from build123d import *
from build123d.topology import SkipClean

# Parameters (mm, degrees)
SKETCH1_R               = 7.9
BOSS_EXTRUDE1_DEPTH     = 1.2
SKETCH2_R               = 1.8
BOSS_EXTRUDE2_DEPTH     = 1.7
CUT_EXTRUDE1_DEPTH      = 12.542530052
CUT_EXTRUDE1_DEPTH_BACK = 12.542530052
SKETCH3_R               = 1.1
BOSS_EXTRUDE3_START     = 2
BOSS_EXTRUDE3_DEPTH     = 2
CUT_EXTRUDE2_DEPTH      = 0.2
CIRPATTERN1_COUNT       = 4
SKETCH6_R               = 1.7
SKETCH6_R_2             = 1.1
BOSS_EXTRUDE4_DEPTH     = 2


with BuildPart() as part:
    # Sketch1 → Boss-Extrude1 (new body)
    with BuildSketch(Plane(origin=(0, 0, 0), x_dir=(1, 0, 0), z_dir=(0, 1, 0))):
        with Locations(Location((0, 0, 0), (0, 0, 270))):
            Circle(SKETCH1_R)
    extrude(amount=BOSS_EXTRUDE1_DEPTH)

    # Sketch2 → Boss-Extrude2 (add)
    with BuildSketch(Plane(origin=(0, 1.2, 0), x_dir=(1, 0, 0), z_dir=(0, 1, 0))):
        with Locations(Location((0, 0, 0), (0, 0, 270))):
            Circle(SKETCH2_R)
    extrude(amount=BOSS_EXTRUDE2_DEPTH)

    # Sketch3 → Cut-Extrude1 (cut, two sides: drawn at the far end of the back side and taken through both)
    with BuildSketch(Plane(origin=(0, 2.9, 0), x_dir=(1, 0, 0), z_dir=(0, 1, 0)).offset(-CUT_EXTRUDE1_DEPTH_BACK)):
        with Locations(Location((0, 0, 0), (0, 0, 270))):
            Circle(SKETCH3_R)
    extrude(amount=CUT_EXTRUDE1_DEPTH + CUT_EXTRUDE1_DEPTH_BACK, mode=Mode.SUBTRACT)

    # Sketch4 → Boss-Extrude3 (add)
    with SkipClean():  # the faces are left unmerged after this step: merging them gives an invalid solid
        with BuildSketch(Plane.XZ.offset(BOSS_EXTRUDE3_START)):
            with BuildLine():
                Line((4.244666906, -6.662792422), (2.951034003, -5.903507289))
                ThreePointArc((2.951034003, -5.903507289), (0, -6.6), (-2.951034003, -5.903507289))
                Line((-2.951034003, -5.903507289), (-4.244666906, -6.662792422))
                ThreePointArc((-4.244666906, -6.662792422), (0, -7.9), (4.244666906, -6.662792422))
            make_face()
        boss_extrude3 = extrude(amount=-BOSS_EXTRUDE3_DEPTH)

    # Sketch5 → Cut-Extrude2 (cut)
    with SkipClean():  # the faces are left unmerged after this step: merging them gives an invalid solid
        with BuildSketch(Plane.XZ.offset(2)):
            with BuildLine():
                Line((-4.050265696, -6.54869054), (-4.244666906, -6.662792422))
                ThreePointArc((-4.244666906, -6.662792422), (0, -7.9), (4.244666906, -6.662792422))
                Line((4.244666906, -6.662792422), (4.050265696, -6.54869054))
                ThreePointArc((4.050265696, -6.54869054), (0, -7.7), (-4.050265696, -6.54869054))
            make_face()
        cut_extrude2 = extrude(amount=-CUT_EXTRUDE2_DEPTH, mode=Mode.SUBTRACT)

    # CirPattern1: Boss-Extrude3, Cut-Extrude2 ×4 about axis
    with SkipClean():  # the faces are left unmerged after this step: merging them gives an invalid solid
        cirpattern1_axis = Axis((0, 0, 0), (0, 1, 0))
        add([boss_extrude3.rotate(cirpattern1_axis, i * 360 / CIRPATTERN1_COUNT) for i in range(1, CIRPATTERN1_COUNT)])
        add([cut_extrude2.rotate(cirpattern1_axis, i * 360 / CIRPATTERN1_COUNT) for i in range(1, CIRPATTERN1_COUNT)], mode=Mode.SUBTRACT)

    # Sketch6 → Boss-Extrude4 (add)
    with SkipClean():  # the faces are left unmerged after this step: merging them gives an invalid solid
        with BuildSketch(Plane.XZ):
            with Locations(Location((0, 0, 0), (0, 0, 90))):
                Circle(SKETCH6_R)
            with Locations(Location((0, 0, 0), (0, 0, 90))):
                Circle(SKETCH6_R_2, mode=Mode.SUBTRACT)
        extrude(amount=BOSS_EXTRUDE4_DEPTH)


solid = part.part
Build history of the part. All positions in model axes, mm. A direction names the side the tool comes from. Round coordinates to 2 decimals unless told otherwise and drop trailing zeros. Write each loop counter-clockwise with the first axis right and the second up, starting at its lowest first coordinate (ties: lowest second). Pieces come first, ordered by that corner, then holes. Notation, with made-up numbers: M 19,70.5 L 61,70.5 A28 cw 61,102.5 Z; hole C -33.75,30 d6. An arc over 180 degrees is marked long. Use CSV: the item, a comma, the result in double quotes.
1. Flat gauge pins, fed straight in: pin 1 (1.5 mm diameter, centred on x = 1, y = 1.5, fed in from -Z); pin 2 (1.8 mm diameter, centred on x = 0, z = 0, fed in from -Y); pin 3 (1 mm diameter, centred on x = 6, z = 5, fed in from -Y). Where does each tip first touch, or does it go through?
Reply:
pin 1,"stops at z = -7.89"
pin 2,"passes through"
pin 3,"stops at y = 0"
2. Saw through at D-D (y = 0.85). Give the cut face in (x, z), plus the area to 3 significant figures.
Reply:
outline,"C 0,0 d15.8; hole C 0,0 d2.2"
area,"192 mm²"
3. Wall check: probe 1 along X at (y, z) = (0.9, 0); probe 2 along X at (y, z) = (-0.85, -0.25); probe 3 along Y at (x, z) = (5.5, 2.75). Give the ranges that are in metal, low to high. Write a range as from..to.
Reply:
probe 1,"x = -7.9..-1.1, 1.1..7.9"
probe 2,"x = -7.9..-6.6, -1.68..-1.07, 1.07..1.68, 6.6..7.9"
probe 3,"y = 0..1.2"
4. Saw through at B-B (z = 0). Give the cut face in (x, y).
Reply:
outline,"M -7.9,-1.8 L -7.7,-1.8 L -7.7,-2 L -6.6,-2 L -6.6,0 L -1.7,0 L -1.7,-2 L -1.1,-2 L -1.1,2.9 L -1.8,2.9 L -1.8,1.2 L -7.9,1.2 Z; M 1.1,-2 L 1.7,-2 L 1.7,0 L 6.6,0 L 6.6,-2 L 7.7,-2 L 7.7,-1.8 L 7.9,-1.8 L 7.9,1.2 L 1.8,1.2 L 1.8,2.9 L 1.1,2.9 Z"
5. Two-plate mould, pull along Y, no slides. Class faces 1 (the face through (1, 2.9, 1)), 2 (the face through (0, -2, 7)), 3 (the face through (-6.28, -1.01, 3.59)): +Y half, -Y half, draft (parallel to the pull), parting line (faces both ways), or undercut.
Reply:
face 1,"+Y half"
face 2,"-Y half"
face 3,"draft"
6. Tool access for faces 4 (the face through (-6.6, -1, 0)), 5 (the face through (6.28, -1.01, -3.59)), 6 (the face through (3.59, -1.01, 6.28)): list every direction of +Z, -Z, +X, -X, +Y, -Y with a clear straight run to the whole face (end or side of a thin tool).
Reply:
face 4,"-Y"
face 5,"-Z, -Y"
face 6,"+X, -Y"
7. Saw through at A-A (y = -0.7). Give the cut face in (x, z).
Reply:
outline,"M -6.66,-4.24 L -5.9,-2.95 A6.6 cw -5.9,2.95 L -6.66,4.24 A7.9 ccw Z; M -4.24,-6.66 A7.9 ccw 4.24,-6.66 L 2.95,-5.9 A6.6 cw -2.95,-5.9 Z; M -4.24,6.66 L -2.95,5.9 A6.6 cw 2.95,5.9 L 4.24,6.66 A7.9 ccw Z; C 0,0 d3.4; M 5.9,-2.95 L 6.66,-4.24 A7.9 ccw 6.66,4.24 L 5.9,2.95 A6.6 cw Z; hole C 0,0 d2.2"
8. Saw through at C-C (x = 0). Give the cut face in (y, z).
Reply:
outline,"M -2,-7.7 L -1.8,-7.7 L -1.8,-7.9 L 1.2,-7.9 L 1.2,-1.8 L 2.9,-1.8 L 2.9,-1.1 L -2,-1.1 L -2,-1.7 L 0,-1.7 L 0,-6.6 L -2,-6.6 Z; M -2,1.1 L 2.9,1.1 L 2.9,1.8 L 1.2,1.8 L 1.2,7.9 L -1.8,7.9 L -1.8,7.7 L -2,7.7 L -2,6.6 L 0,6.6 L 0,1.7 L -2,1.7 Z"
